```python
from build123d import *

# Parameters (mm, degrees)
SKETCH1_W           = 15
SKETCH1_H           = 13
BOSS_EXTRUDE1_DEPTH = 1
SKETCH2_R           = 0.875
BOSS_EXTRUDE2_DEPTH = 7.5
SKETCH3_W           = 5
SKETCH3_H           = 5
CUT_EXTRUDE1_DEPTH  = 10
SKETCH4_R           = 0.5
CUT_EXTRUDE2_DEPTH  = 2


with BuildPart() as part:
    # Sketch1 → Boss-Extrude1 (new body)
    with BuildSketch(Plane(origin=(0, 0, 0), x_dir=(1, 0, 0), z_dir=(0, 1, 0))):
        with Locations((10.569631841, -166.54341444)):
            Rectangle(SKETCH1_W, SKETCH1_H)
    extrude(amount=BOSS_EXTRUDE1_DEPTH)

    # Sketch2 → Boss-Extrude2 (add)
    with BuildSketch(Plane(origin=(18.069631841, 0, 0), x_dir=(0, 0, -1), z_dir=(1, 0, 0))):
        with Locations((-173.04341444, 0.875)):
            Circle(SKETCH2_R)
    extrude(amount=-BOSS_EXTRUDE2_DEPTH)

    # Sketch3 → Cut-Extrude1 (cut)
    with BuildSketch(Plane(origin=(0, 0, 0), x_dir=(-1, 0, 0), z_dir=(0, -1, 0))):
        with Locations((-10.569631841, -162.54341444)):
            Rectangle(SKETCH3_W, SKETCH3_H)
    extrude(amount=-CUT_EXTRUDE1_DEPTH, mode=Mode.SUBTRACT)

    # Sketch4 → Cut-Extrude2 (cut, through all)
    with BuildSketch(Plane(origin=(0, 1, 0), x_dir=(1, 0, 0), z_dir=(0, 1, 0))):
        with Locations((15.569631841, -162.54341444)):
            Circle(SKETCH4_R)
        with Locations((15.569631841, -170.04341444)):
            Circle(SKETCH4_R)
        with Locations((10.569631841, -170.04341444)):
            Circle(SKETCH4_R)
        with Locations((5.569631841, -170.04341444)):
            Circle(SKETCH4_R)
        with Locations((5.569631841, -162.54341444)):
            Circle(SKETCH4_R)
    extrude(amount=-CUT_EXTRUDE2_DEPTH, mode=Mode.SUBTRACT)


solid = part.part
```
Could you check a few things on this model? Use its own coordinates, in mm. A direction names the side the tool comes from. Round coordinates to 2 decimals unless told otherwise and drop trailing zeros. Loops run counter-clockwise (first coordinate to the right, second up) from the corner with the lowest first, then second, coordinate; pieces in that order, holes last. Notation, with made-up numbers: (75.25, 78) - (92.25, 78) arc R19 cw to (92.25, 98) - close; hole circle Ø8 at (35.25, -29). An arc over 180 degrees is marked (long way). Answer in a Markdown table with one row per item. Add a question column.
(1) If we section it at B-B (y = 0.25): Please give me the cut outline in (x, z), plus the area to 3 significant figures.
(2) If we section it at A-A (z = 161): Please give me the cut outline in (x, y), plus the area to 3 significant figures.
(3) If we section it at D-D (x = 12.5): Please give me the cut outline in (y, z) (3 decimals).
(4) I'm going to push a flat-ended pin straight in: pin 1 (8 mm diameter, centred on x = 9.5, z = 162.5, fed in from +Y). Where does the tip first touch, or does it pass through?
(5) If we section it at C-C (x = 5.25): Please give me the cut outline in (y, z), plus the area to 3 significant figures.
(6) For faces 1 (the face through (6.8, 0.5, 173.043)), 2 (the face through (13.07, 0.5, 162.6)), 3 (the face through (5.5, 0.5, 160.043)), which set-ups out of +Z, -Z, +X, -X, +Y, -Y let a thin tool reach every point of the face, with its end or its side?
(7) I need wall thicknesses on line 1 along X through (y, z) = (0.15, 170); line 2 along X through (y, z) = (0.35, 161.25); line 3 along X through (y, z) = (0.35, 169.75). Which ranges of each line are inside material? Lowest first, please.
(8) If we mould it in two halves opening along X, with no side actions, what happens to faces 4 (the face through (10.5, 0.51, 169.55)), 5 (the face through (18.07, 0.5, 167.1)), 6 (the face through (10, 0, 168))? For each: pulls with the +X half, pulls with the -X half, needs draft (parallel to the pull), parting line crosses it, or undercut.
Model answer:
| question | item | result |
|---|---|---|
| 1 | outline | (3.07, 160.04) - (8.07, 160.04) - (8.07, 165.04) - (13.07, 165.04) - (13.07, 160.04) - (18.07, 160.04) - (18.07, 173.66) - (10.57, 173.66) - (10.57, 173.04) - (3.07, 173.04) - close; hole circle Ø1 at (5.57, 162.54); hole circle Ø1 at (5.57, 170.04); hole circle Ø1 at (10.57, 170.04); hole circle Ø1 at (15.57, 162.54); hole circle Ø1 at (15.57, 170.04) |
| 1 | area | 171 mm² |
| 2 | outline | (3.07, 0) - (8.07, 0) - (8.07, 1) - (3.07, 1) - close; (13.07, 0) - (18.07, 0) - (18.07, 1) - (13.07, 1) - close |
| 2 | area | 10.0 mm² |
| 3 | outline | (0, 165.043) - (1, 165.043) - (1, 172.177) arc R0.875 ccw (long way) to (0, 173.043) - close |
| 4 | pin 1 | stops at y = 1 |
| 5 | outline | (0, 160.04) - (1, 160.04) - (1, 162.16) - (0, 162.16) - close; (0, 162.93) - (1, 162.93) - (1, 169.66) - (0, 169.66) - close; (0, 170.43) - (1, 170.43) - (1, 173.04) - (0, 173.04) - close |
| 5 | area | 11.5 mm² |
| 6 | face 1 | +Z, -X, +Y, -Y |
| 6 | face 2 | -Z, +Y, -Y |
| 6 | face 3 | -Z, +X, -X, +Y, -Y |
| 7 | line 1 | x = 3.07 to 5.07, 6.07 to 10.07, 11.07 to 15.07, 16.07 to 18.07 |
| 7 | line 2 | x = 3.07 to 8.07, 13.07 to 18.07 |
| 7 | line 3 | x = 3.07 to 5.16, 5.97 to 10.16, 10.97 to 15.16, 15.97 to 18.07 |
| 8 | face 4 | undercut |
| 8 | face 5 | pulls with the +X half |
| 8 | face 6 | needs draft |
